Answer from the drawing. Dimensions are ordinates in mm from the lowest x, y and z of the part. A direction names the side the tool comes from. Give positions to 0.01 mm unless a question says otherwise; leave off trailing zeros. Order: outer loops, then holes, each group sorted by start corner. A loop starts at its lowest first (then second) coordinate and runs counter-clockwise, first axis right, second up. Notation, with made-up numbers: (23.25, -28.5) - (80.25, -28.5) arc R27 ccw to (80.25, 0.5) - close; hole circle Ø7 at (12, -19). An arc over 180 degrees is marked (long way). Answer in a Markdown table with one row per item. Add a question column.
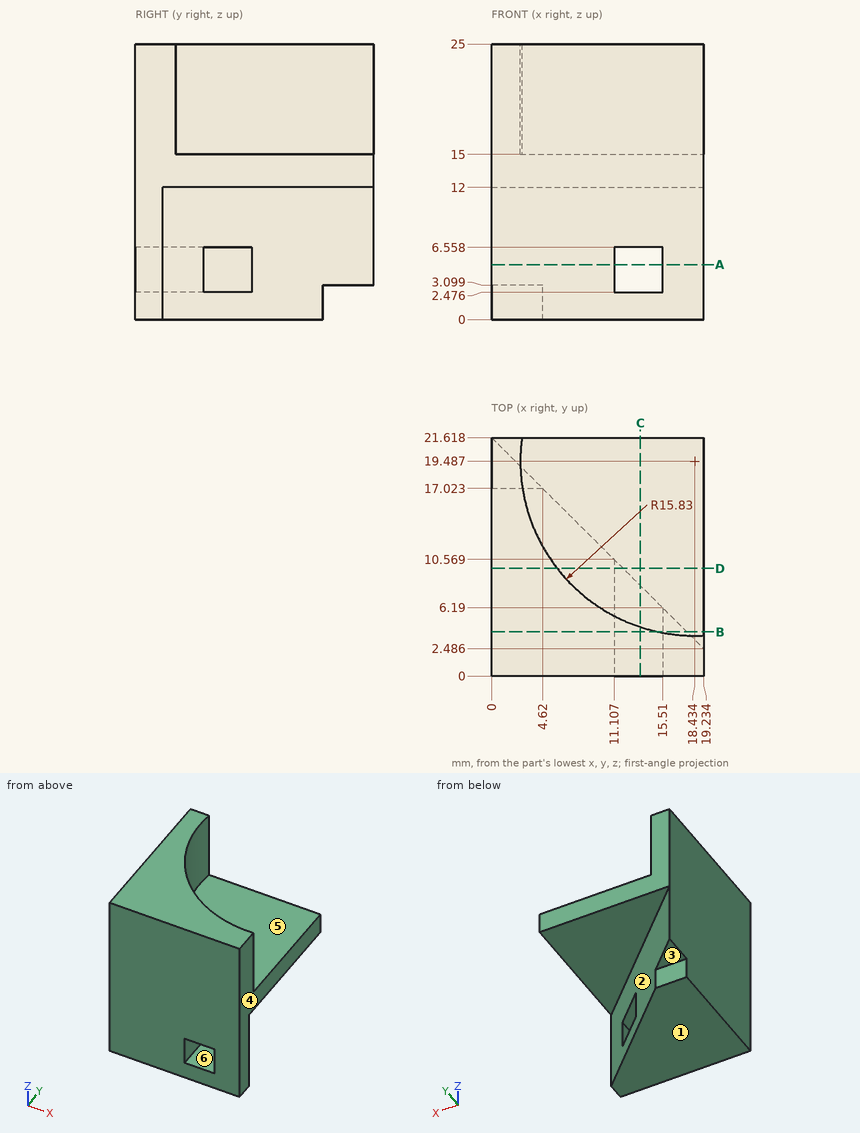
(1) Straight lines are drawn through the part: line 1 (Z direction, x = 13.5, y = 7); line 2 (Z direction, x = 13.5, y = 1.75); line 3 (Z direction, x = 18.75, y = 17.5). For each, find the intervals that lie inside material, in ascending order.
(2) Find section B-B, the plane y = 4. Write down the section's boundary in (x, z) (1 decimal).
(3) Find section C-C, the plane x = 13.5. Write down the section's boundary in (y, z) (1 decimal).
(4) The mould has two halves that part along X. Classify the marked faces 4, 5 and 6: +X half, -X half, draft (parallel to the pull), parting line (faces both ways), or undercut.
(5) Find section A-A, the plane z = 5. Write down the section's boundary in (x, y) (1 decimal).
(6) For the marked faces 1, 2 and 3, determine the directions among +Z, -Z, +X, -X, +Y, -Y from which every point of the face is accessible in a straight line to the end or side of a thin tool.
(7) Find section D-D, the plane y = 9.75. Write down the section's boundary in (x, z), plus the area to 3 significant figures.
(8) Each of these flat-tipped pins is pushed along its axis until it touches: P1, Ø1.5, axis at x = 8.5, z = 9.5, coming from the +Y side; P2, Ø8.5, axis at x = 15, y = 14.5, coming from the +Z side; P3, Ø4, axis at y = 19, z = 3.5, coming from the +X side. Where does it stop, or does it pass through?
Answer key:
| question | item | result |
|---|---|---|
| 1 | line 1 | 0 to 2.48, 6.56 to 15 |
| 1 | line 2 | 0 to 2.48, 6.56 to 25 |
| 1 | line 3 | 12 to 15 |
| 2 | outline | (0, 0) - (17.7, 0) - (17.7, 12) - (19.2, 12) - (19.2, 15) - (15.2, 15) - (15.2, 25) - (0, 25) - close; hole (11.1, 2.5) - (15.5, 2.5) - (15.5, 6.6) - (11.1, 6.6) - close |
| 3 | outline | (0, 0) - (8.2, 0) - (8.2, 2.5) - (0, 2.5) - close; (0, 6.6) - (8.2, 6.6) - (8.2, 12) - (21.6, 12) - (21.6, 15) - (4.4, 15) - (4.4, 25) - (0, 25) - close |
| 4 | face 4 | +X half |
| 4 | face 5 | draft |
| 4 | face 6 | undercut |
| 5 | outline | (0, 0) - (11.1, 0) - (11.1, 10.6) - (0, 21.6) - close; (15.5, 0) - (19.2, 0) - (19.2, 2.5) - (15.5, 6.2) - close |
| 6 | face 1 | -Z, +X, -X, +Y, -Y |
| 6 | face 2 | -Z, +X, +Y |
| 6 | face 3 | -Z, +X, -X, +Y |
| 7 | outline | (0, 0) - (11.93, 0) - (11.93, 2.48) - (11.11, 2.48) - (11.11, 6.56) - (11.93, 6.56) - (11.93, 12) - (19.23, 12) - (19.23, 15) - (5.95, 15) - (5.95, 25) - (0, 25) - close |
| 7 | area | 257 mm² |
| 8 | P1 | y = 13.91 |
| 8 | P2 | z = 15 |
| 8 | P3 | x = 4.64 |
